Work out the finished part from the listing and answer in its coordinate system (mm). Give positions to 0.01 mm unless a question says otherwise; leave off trailing zeros. Loops run counter-clockwise (first coordinate to the right, second up) from the corner with the lowest first, then second, coordinate; pieces in that order, holes last. Notation, with made-up numbers: M 72.5,33 L 80.5,33 A10 cw 80.5,51 Z; hole C 87.5,-3.75 d8. An arc over 180 degrees is marked long. Use a Markdown table: item, result.
```python
from build123d import *

# Parameters (mm, degrees)
SKETCH1_R           = 3.175
BOSS_EXTRUDE1_DEPTH = 3.175
SKETCH2_R           = 11.049
SKETCH2_R_2         = 15.875
SKETCH2_R_3         = 1.27
CUT_EXTRUDE1_DEPTH  = 202.930998425
SKETCH3_W           = 38.1
SKETCH3_H           = 6.35
SKETCH3_W_2         = 88.9
CUT_EXTRUDE4_DEPTH  = 202.930998425
CUT_EXTRUDE5_DEPTH  = 202.930998425
SKETCH5_R           = 2.003539073
SKETCH5_R_2         = 2.332520908
CUT_EXTRUDE6_DEPTH  = 202.930998425
SKETCH6_R           = 1.5875
CUT_EXTRUDE7_DEPTH  = 202.930998425
SKETCH7_R           = 1.5875
CUT_EXTRUDE8_DEPTH  = 202.930998425


with BuildPart() as part:
    # Sketch1 → Boss-Extrude1 (new, symmetric)
    with BuildSketch(Plane.XY):
        with BuildLine():
            Line((-145.783553311, 66.675), (145.783553311, 66.675))
            ThreePointArc((145.783553311, 66.675), (147.900219978, 66.497368874), (149.957676269, 65.969444444))
            ThreePointArc((149.957676269, 65.969444444), (172.789871953, 52.74760778), (189.088888889, 31.999880883))
            ThreePointArc((189.088888889, 31.999880883), (190.142181511, 29.17513943), (190.5, 26.181720723))
            Line((190.5, 26.181720723), (190.5, -22.225))
            ThreePointArc((190.5, -22.225), (186.780256121, -31.205256121), (177.8, -34.925))
            Line((177.8, -34.925), (-177.8, -34.925))
            ThreePointArc((-177.8, -34.925), (-186.780256121, -31.205256121), (-190.5, -22.225))
            Line((-190.5, -22.225), (-190.5, 26.181720723))
            ThreePointArc((-190.5, 26.181720723), (-190.142181511, 29.17513943), (-189.088888889, 31.999880883))
            ThreePointArc((-189.088888889, 31.999880883), (-172.789871953, 52.74760778), (-149.957676269, 65.969444444))
            ThreePointArc((-149.957676269, 65.969444444), (-147.900219978, 66.497368874), (-145.783553311, 66.675))
        make_face()
        with Locations((-127, 0)):
            Circle(SKETCH1_R, mode=Mode.SUBTRACT)
        with Locations((127, 0)):
            Circle(SKETCH1_R, mode=Mode.SUBTRACT)
    extrude(amount=BOSS_EXTRUDE1_DEPTH, both=True)

    # Sketch2 → Cut-Extrude1 (cut, through all)
    with BuildSketch(Plane.XY.offset(3.175)):
        with Locations((-127, 0)):
            Circle(SKETCH2_R)
        with Locations((-155.575, 0)):
            Circle(SKETCH2_R_2)
        with Locations((-155.575, 23.8125)):
            Circle(SKETCH2_R_3)
        with Locations((-138.737019773, 16.837980227)):
            Circle(SKETCH2_R_3)
        with Locations((-138.737019773, -16.837980227)):
            Circle(SKETCH2_R_3)
        with Locations((-155.575, -23.8125)):
            Circle(SKETCH2_R_3)
        with Locations((-172.412980227, -16.837980227)):
            Circle(SKETCH2_R_3)
        with Locations((-179.3875, 0)):
            Circle(SKETCH2_R_3)
        with Locations((-172.412980227, 16.837980227)):
            Circle(SKETCH2_R_3)
        with Locations((-127, 15.875)):
            Circle(SKETCH2_R_3)
        with Locations((-115.774679849, 11.225320151)):
            Circle(SKETCH2_R_3)
        with Locations((-111.125, 0)):
            Circle(SKETCH2_R_3)
        with Locations((-115.774679849, -11.225320151)):
            Circle(SKETCH2_R_3)
        with Locations((-127, -15.875)):
            Circle(SKETCH2_R_3)
        with Locations((-138.225320151, -11.225320151)):
            Circle(SKETCH2_R_3)
        with Locations(Location((138.225320151, 11.225320151, 0), (0, 0, 180))):
            Circle(SKETCH2_R_3)
        with Locations((-138.225320151, 11.225320151)):
            Circle(SKETCH2_R_3)
        with Locations(Location((138.225320151, -11.225320151, 0), (0, 0, 180))):
            Circle(SKETCH2_R_3)
        with Locations(Location((127, -15.875, 0), (0, 0, 180))):
            Circle(SKETCH2_R_3)
        with Locations(Location((115.774679849, -11.225320151, 0), (0, 0, 180))):
            Circle(SKETCH2_R_3)
        with Locations(Location((111.125, 0, 0), (0, 0, 180))):
            Circle(SKETCH2_R_3)
        with Locations(Location((115.774679849, 11.225320151, 0), (0, 0, 180))):
            Circle(SKETCH2_R_3)
        with Locations(Location((127, 15.875, 0), (0, 0, 180))):
            Circle(SKETCH2_R_3)
        with Locations(Location((172.412980227, 16.837980227, 0), (0, 0, 180))):
            Circle(SKETCH2_R_3)
        with Locations(Location((179.3875, 0, 0), (0, 0, 180))):
            Circle(SKETCH2_R_3)
        with Locations(Location((172.412980227, -16.837980227, 0), (0, 0, 180))):
            Circle(SKETCH2_R_3)
        with Locations(Location((155.575, -23.8125, 0), (0, 0, 180))):
            Circle(SKETCH2_R_3)
        with Locations(Location((138.737019773, -16.837980227, 0), (0, 0, 180))):
            Circle(SKETCH2_R_3)
        with Locations(Location((138.737019773, 16.837980227, 0), (0, 0, 180))):
            Circle(SKETCH2_R_3)
        with Locations(Location((155.575, 23.8125, 0), (0, 0, 180))):
            Circle(SKETCH2_R_3)
        with Locations(Location((155.575, 0, 0), (0, 0, 180))):
            Circle(SKETCH2_R_2)
        with Locations(Location((127, 0, 0), (0, 0, 180))):
            Circle(SKETCH2_R)
    extrude(amount=-CUT_EXTRUDE1_DEPTH, mode=Mode.SUBTRACT)

    # Sketch3 → Cut-Extrude4 (cut, through all)
    with BuildSketch(Plane.XY.offset(3.175)):
        with Locations((-120.383553311, 63.5)):
            Rectangle(SKETCH3_W, SKETCH3_H)
        with Locations((120.383553311, 63.5)):
            Rectangle(SKETCH3_W, SKETCH3_H)
        with Locations((0, 63.5)):
            Rectangle(SKETCH3_W_2, SKETCH3_H)
    extrude(amount=-CUT_EXTRUDE4_DEPTH, mode=Mode.SUBTRACT)

    # Sketch4 → Cut-Extrude5 (cut, through all)
    with BuildSketch(Plane.XY.offset(3.175)):
        with BuildLine():
            Line((-63.5, 41.275), (-22.225, 41.275))
            ThreePointArc((-22.225, 41.275), (-13.244743879, 37.555256121), (-9.525, 28.575))
            Line((-9.525, 28.575), (-9.525, -3.175))
            ThreePointArc((-9.525, -3.175), (-13.244743879, -12.155256121), (-22.225, -15.875))
            Line((-22.225, -15.875), (-63.5, -15.875))
            ThreePointArc((-63.5, -15.875), (-72.480256121, -12.155256121), (-76.2, -3.175))
            Line((-76.2, -3.175), (-76.2, 28.575))
            ThreePointArc((-76.2, 28.575), (-72.480256121, 37.555256121), (-63.5, 41.275))
        make_face()
        with BuildLine():
            Line((76.2, 28.575), (76.2, -3.175))
            ThreePointArc((76.2, -3.175), (72.480256121, -12.155256121), (63.5, -15.875))
            Line((63.5, -15.875), (22.225, -15.875))
            ThreePointArc((22.225, -15.875), (13.244743879, -12.155256121), (9.525, -3.175))
            Line((9.525, -3.175), (9.525, 28.575))
            ThreePointArc((9.525, 28.575), (13.244743879, 37.555256121), (22.225, 41.275))
            Line((22.225, 41.275), (63.5, 41.275))
            ThreePointArc((63.5, 41.275), (72.480256121, 37.555256121), (76.2, 28.575))
        make_face()
    extrude(amount=-CUT_EXTRUDE5_DEPTH, mode=Mode.SUBTRACT)

    # Sketch5 → Cut-Extrude6 (cut, through all)
    with BuildSketch(Plane.XY.offset(3.175)):
        with Locations((-135.306053311, 53.975)):
            Circle(SKETCH5_R)
        with Locations(Location((-105.461053311, 53.975, 0), (0, 0, 180))):
            Circle(SKETCH5_R)
        with Locations((105.461053311, 53.975)):
            Circle(SKETCH5_R)
        with Locations(Location((135.306053311, 53.975, 0), (0, 0, 180))):
            Circle(SKETCH5_R)
        with Locations((-14.9225, 53.975)):
            Circle(SKETCH5_R_2)
        with Locations(Location((14.9225, 53.975, 0), (0, 0, 180))):
            Circle(SKETCH5_R_2)
    extrude(amount=-CUT_EXTRUDE6_DEPTH, mode=Mode.SUBTRACT)

    # Sketch6 → Cut-Extrude7 (cut, through all)
    with BuildSketch(Plane.XY.offset(3.175)):
        with Locations((-177.8, -28.575)):
            Circle(SKETCH6_R)
        with Locations((-107.95, -28.575)):
            Circle(SKETCH6_R)
        with Locations(Location((107.95, -28.575, 0), (0, 0, 180))):
            Circle(SKETCH6_R)
        with Locations(Location((177.8, -28.575, 0), (0, 0, 180))):
            Circle(SKETCH6_R)
    extrude(amount=-CUT_EXTRUDE7_DEPTH, mode=Mode.SUBTRACT)

    # Sketch7 → Cut-Extrude8 (cut, through all)
    with BuildSketch(Plane.XY.offset(3.175)):
        Circle(SKETCH7_R)
    extrude(amount=-CUT_EXTRUDE8_DEPTH, mode=Mode.SUBTRACT)


solid = part.part
```
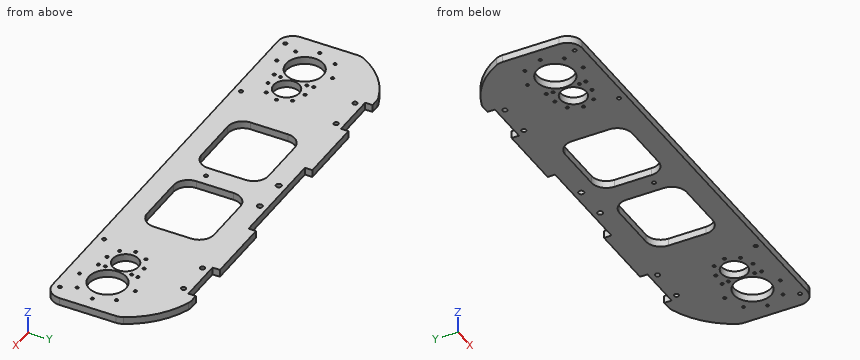
(1) A cutting plane is placed at A-A (x = 68). Write down the section's boundary in (y, z) (3 decimals).
Entries:
| item | result |
|---|---|
| outline | M -34.925,-3.175 L -15.051,-3.175 L -15.051,3.175 L -34.925,3.175 Z; M 40.451,-3.175 L 66.675,-3.175 L 66.675,3.175 L 40.451,3.175 Z |
(2) Given P1, Ø8, axis at x = -47.5, y = -9.5, coming from the +Z side; P2, Ø1.9, axis at y = 62.5, z = 1.5, coming from the -X side; P3, Ø1.9, axis at y = 62, z = -1, coming from the +X side, each flat-ended and moving along its own axis, determine where each tip first touches the part or whether it passes through.
Entries:
| item | result |
|---|---|
| P1 | passes through |
| P2 | stops at x = -160.02 |
| P3 | stops at x = 160.94 |
(3) Consider probe 1 along X at (y, z) = (19.5, 2) (3 decimals); probe 2 along X at (y, z) = (23.5, 0.5) (3 decimals); probe 3 along X at (y, z) = (34, 2.5). Determine where each line is inside the solid, lowest interval first. Write a range as [from, to].
Entries:
| item | result |
|---|---|
| probe 1 | x = [-190.5, -76.2], [-9.525, 9.525], [76.2, 190.5] |
| probe 2 | x = [-190.5, -156.806], [-154.344, -76.2], [-9.525, 9.525], [76.2, 154.344], [156.806, 190.5] |
| probe 3 | x = [-188.02, -74.98], [-10.74, 10.74], [74.98, 188.02] |
(4) A cutting plane is placed at B-B (z = -1.5). Count the separate pieces of the cut face and the enclosed holes in it, and give its area (3 significant figures).
Entries:
| item | result |
|---|---|
| separate pieces | 1 |
| enclosed holes | 45 |
| area | 26,500 mm² |
